Here's how the part is built. I have some questions about the finished solid (model axes, mm). A direction names the side the tool comes from. Coordinates: 2 decimals unless noted, no trailing zeros. Loops run counter-clockwise (first coordinate to the right, second up) from the corner with the lowest first, then second, coordinate; pieces in that order, holes last. Notation, with made-up numbers: (71, 40.25) -> (129, 40.25) arc R27 ccw to (129, 74.25) -> close; hole circle Ø5 at (-27.5, 3.5). An arc over 180 degrees is marked (long way). Answer as a JSON object with one key per item and string values. Group by question number.
Q1. Thinking about a two-plate mould opening in Z: for faces 3 (the flat face through (-1, 3, 21.209)), 4 (the flat face through (16, 3, 8.509)), 5 (the flat face through (-19.05, 3, -12)), 6 (the flat face through (-44.45, 3, 0)), which applies, released by +Z, released by -Z, zero draft, split by the parting line, or undercut?
Q2. I want a section at A-A on z = -11. Write out the boundary of the cut face in (x, y).
Q3. I want a section at C-C on y = 4. Count the separate pieces of the cut face and the enclosed holes in it, then the cut area to 3 significant figures.
Q4. I need wall thicknesses on line 1 (Z direction, x = -16, y = 1.75); line 2 (X direction, y = 5, z = 0); line 3 (X direction, y = 2.75, z = 13). Which ranges of each line are inside material? Lowest first, please.
Q5. I want a section at B-B on z = 0. Write out the boundary of the cut face in (x, y).
Q6. On a 3-axis mill with a long thin cutter (end or side, diameter ignored), from which of +Z, -Z, +X, -X, +Y, -Y can I reach the whole of each face in a straight line? I mean faces 1 (the flat face through (-19.05, 3, 12)), 2 (the flat face through (44.45, 3, 0)). Say none if no direction works.
```python
from build123d import *

# Parameters (mm, degrees)
ELEVATOR_SPACER_W   = 88.9
ELEVATOR_SPACER_H   = 42.418
ELEVATOR_SPACER_R   = 2.159
ELEVATOR_SPACER_W_2 = 6.35
ELEVATOR_SPACER_H_2 = 6.35
BOSS_EXTRUDE1_DEPTH = 6.35


with BuildPart() as part:
    # Elevator Spacer → Boss-Extrude1 (new body)
    with BuildSketch(Plane(origin=(0, 0, 0), x_dir=(1, 0, 0), z_dir=(0, 1, 0))):
        Rectangle(ELEVATOR_SPACER_W, ELEVATOR_SPACER_H)
        with Locations(Location((34.925, 0, 0), (0, 0, 270))):
            Circle(ELEVATOR_SPACER_R, mode=Mode.SUBTRACT)
        with Locations(Location((15.875, 0, 0), (0, 0, 270))):
            Circle(ELEVATOR_SPACER_R, mode=Mode.SUBTRACT)
        with Locations(Location((-15.875, 0, 0), (0, 0, 90))):
            Circle(ELEVATOR_SPACER_R, mode=Mode.SUBTRACT)
        with Locations(Location((-34.925, 0, 0), (0, 0, 90))):
            Circle(ELEVATOR_SPACER_R, mode=Mode.SUBTRACT)
        with Locations((34.925, 11.684)):
            Rectangle(ELEVATOR_SPACER_W_2, ELEVATOR_SPACER_H_2, mode=Mode.SUBTRACT)
        with Locations((34.925, -11.684)):
            Rectangle(ELEVATOR_SPACER_W_2, ELEVATOR_SPACER_H_2, mode=Mode.SUBTRACT)
        with Locations((15.875, 11.684)):
            Rectangle(ELEVATOR_SPACER_W_2, ELEVATOR_SPACER_H_2, mode=Mode.SUBTRACT)
        with Locations((15.875, -11.684)):
            Rectangle(ELEVATOR_SPACER_W_2, ELEVATOR_SPACER_H_2, mode=Mode.SUBTRACT)
        with Locations((-15.875, -11.684)):
            Rectangle(ELEVATOR_SPACER_W_2, ELEVATOR_SPACER_H_2, mode=Mode.SUBTRACT)
        with Locations((-15.875, 11.684)):
            Rectangle(ELEVATOR_SPACER_W_2, ELEVATOR_SPACER_H_2, mode=Mode.SUBTRACT)
        with Locations((-34.925, -11.684)):
            Rectangle(ELEVATOR_SPACER_W_2, ELEVATOR_SPACER_H_2, mode=Mode.SUBTRACT)
        with Locations((-34.925, 11.684)):
            Rectangle(ELEVATOR_SPACER_W_2, ELEVATOR_SPACER_H_2, mode=Mode.SUBTRACT)
    extrude(amount=BOSS_EXTRUDE1_DEPTH)


solid = part.part
```
Result set:
{
 "1": {"face 3": "released by +Z", "face 4": "undercut", "face 5": "undercut", "face 6": "zero draft"},
 "2": {"outline": "(-44.45, 0) -> (-38.1, 0) -> (-38.1, 6.35) -> (-44.45, 6.35) -> close; (-31.75, 0) -> (-19.05, 0) -> (-19.05, 6.35) -> (-31.75, 6.35) -> close; (-12.7, 0) -> (12.7, 0) -> (12.7, 6.35) -> (-12.7, 6.35) -> close; (19.05, 0) -> (31.75, 0) -> (31.75, 6.35) -> (19.05, 6.35) -> close; (38.1, 0) -> (44.45, 0) -> (44.45, 6.35) -> (38.1, 6.35) -> close"},
 "3": {"separate pieces": "1", "enclosed holes": "12", "area": "3,390 mm²"},
 "4": {"line 1": "z = -21.21 to -14.86, -8.51 to -2.16, 2.16 to 8.51, 14.86 to 21.21", "line 2": "x = -44.45 to -37.08, -32.77 to -18.03, -13.72 to 13.72, 18.03 to 32.77, 37.08 to 44.45", "line 3": "x = -44.45 to -38.1, -31.75 to -19.05, -12.7 to 12.7, 19.05 to 31.75, 38.1 to 44.45"},
 "5": {"outline": "(-44.45, 0) -> (-37.08, 0) -> (-37.08, 6.35) -> (-44.45, 6.35) -> close; (-32.77, 0) -> (-18.03, 0) -> (-18.03, 6.35) -> (-32.77, 6.35) -> close; (-13.72, 0) -> (13.72, 0) -> (13.72, 6.35) -> (-13.72, 6.35) -> close; (18.03, 0) -> (32.77, 0) -> (32.77, 6.35) -> (18.03, 6.35) -> close; (37.08, 0) -> (44.45, 0) -> (44.45, 6.35) -> (37.08, 6.35) -> close"},
 "6": {"face 1": "+Y, -Y", "face 2": "+Z, -Z, +X, +Y, -Y"}
}
